Input: part model. Units: mm. Frame: model coordinates. A direction names the side the tool comes from. Give positions to 0.01 mm unless a question says otherwise; leave off trailing zeros. Order: outer loops, then holes, each group sorted by start corner. A loop starts at its lowest first (then second) coordinate and runs counter-clockwise, first axis right, second up. Notation, with made-up numbers: (-20.75, 75) - (16.25, 75) arc R33 cw to (16.25, 104) - close; hole circle Ø11 at (55, -38). An arc over 180 degrees is marked (long way). Answer in a Markdown table with one row per item. Add a question column.
1. Ray query, line 1 (Y direction, x = 90.5, z = 0.55); line 2 (X direction, y = 67.5, z = 0.6); line 3 (X direction, y = 45, z = 5.5). Return the intervals inside material, ascending. Write a range as [from, to].
2. Access query for faces 5 (the face through (46, 9.5, 6)), 6 (the face through (7.5, 35, 6)), 7 (the face through (85.5, 35, 6)), 8 (the face through (40, 3.6, -4)), 9 (the face through (65, 2, -4)). Directions: +Z, -Z, +X, -X, +Y, -Y. A direction counts if a zero-diameter tool reaches every point of the face in a straight line with its end or side. Return the directions, or none.
3. Section query C-C on x = 81. Return loops of the section in (y, z).
4. Contact query for flat-ended pins moving along their axis: pin 1 (5 mm diameter, centred on x = 2.5, y = 2.5, fed in from +Z); pin 2 (2.5 mm diameter, centred on x = 51.5, z = -3.5, fed in from +Y); pin 3 (1.5 mm diameter, centred on x = 79.5, y = 33.5, fed in from -Z); pin 4 (9 mm diameter, centred on x = 35, z = -3.5, fed in from -Y). Output: stop coordinate, or through.
5. Mould query, pull axis X, two halves, no side actions, for faces 1 (the face through (14, 2, -4)), 2 (the face through (40, 1.4, -4)), 3 (the face through (3.306, 68.765, 0.811)), 4 (the face through (40, 3, -8)). Classes: released by +X, released by -X, zero draft, split by the parting line, or undercut.
6. Section query D-D on y = 8. Return loops of the section in (x, z), and give its area (3 significant figures).
7. Section query A-A on x = 90.5. Return loops of the section in (y, z).
8. Section query B-B on y = 40. Return loops of the section in (x, z).
```python
from build123d import *

# Parameters (mm, degrees)
SKETCH_1_W          = 93
SKETCH_1_H          = 70
EXTRUDE_1_DEPTH     = 1.6
SKETCH_2_R          = 1.5
CUT_EXTRUDE_1_DEPTH = 117.411167849
SKETCH_3_W          = 78
SKETCH_3_H          = 51
EXTRUDE_2_DEPTH     = 9
SKETCH_4_W          = 51
SKETCH_4_H          = 2.2
EXTRUDE_3_DEPTH     = 8
SKETCH_5_R          = 0.4
EXTRUDE_4_DEPTH     = 2


with BuildPart() as part:
    # 草图1 → 凸台-拉伸1 (new body)
    with BuildSketch(Plane.XY):
        with Locations((46.5, 35)):
            Rectangle(SKETCH_1_W, SKETCH_1_H)
    extrude(amount=EXTRUDE_1_DEPTH)

    # 草图2 → 切除-拉伸1 (cut, through all)
    with BuildSketch(Plane.XY.offset(1.6)):
        with Locations((2.5, 2.5)):
            Circle(SKETCH_2_R)
        with Locations((90.5, 2.5)):
            Circle(SKETCH_2_R)
        with Locations((90.5, 67.5)):
            Circle(SKETCH_2_R)
        with Locations((2.5, 67.5)):
            Circle(SKETCH_2_R)
    extrude(amount=-CUT_EXTRUDE_1_DEPTH, mode=Mode.SUBTRACT)

    # 草图3 → 凸台-拉伸2 (add)
    with BuildSketch(Plane.XY.offset(1.6)):
        with Locations((46.5, 35)):
            Rectangle(SKETCH_3_W, SKETCH_3_H)
    extrude(amount=EXTRUDE_2_DEPTH)

    # 草图4 → 凸台-拉伸3 (add)
    with BuildSketch(Plane(origin=(0, 0, 0), x_dir=(-1, 0, 0), z_dir=(0, 0, -1))):
        with Locations((-39.5, 2.5)):
            Rectangle(SKETCH_4_W, SKETCH_4_H)
    extrude(amount=EXTRUDE_3_DEPTH)

    # 草图5 → 凸台-拉伸4 (add)
    with BuildSketch(Plane(origin=(0, 0, -8), x_dir=(-1, 0, 0), z_dir=(0, 0, -1))):
        with Locations(Location((-38.23, 2.5, 0), (0, 0, 180))):
            Circle(SKETCH_5_R)
        with Locations(Location((-40.77, 2.5, 0), (0, 0, 180))):
            Circle(SKETCH_5_R)
        with Locations(Location((-43.31, 2.5, 0), (0, 0, 180))):
            Circle(SKETCH_5_R)
        with Locations(Location((-45.85, 2.5, 0), (0, 0, 180))):
            Circle(SKETCH_5_R)
        with Locations(Location((-48.39, 2.5, 0), (0, 0, 180))):
            Circle(SKETCH_5_R)
        with Locations(Location((-50.93, 2.5, 0), (0, 0, 180))):
            Circle(SKETCH_5_R)
        with Locations(Location((-53.47, 2.5, 0), (0, 0, 180))):
            Circle(SKETCH_5_R)
        with Locations(Location((-56.01, 2.5, 0), (0, 0, 180))):
            Circle(SKETCH_5_R)
        with Locations(Location((-58.55, 2.5, 0), (0, 0, 180))):
            Circle(SKETCH_5_R)
        with Locations(Location((-61.09, 2.5, 0), (0, 0, 180))):
            Circle(SKETCH_5_R)
        with Locations(Location((-63.63, 2.5, 0), (0, 0, 180))):
            Circle(SKETCH_5_R)
        with Locations(Location((-35.69, 2.5, 0), (0, 0, 180))):
            Circle(SKETCH_5_R)
        with Locations(Location((-33.15, 2.5, 0), (0, 0, 180))):
            Circle(SKETCH_5_R)
        with Locations(Location((-30.61, 2.5, 0), (0, 0, 180))):
            Circle(SKETCH_5_R)
        with Locations(Location((-28.07, 2.5, 0), (0, 0, 180))):
            Circle(SKETCH_5_R)
        with Locations(Location((-25.53, 2.5, 0), (0, 0, 180))):
            Circle(SKETCH_5_R)
        with Locations(Location((-22.99, 2.5, 0), (0, 0, 180))):
            Circle(SKETCH_5_R)
        with Locations(Location((-20.45, 2.5, 0), (0, 0, 180))):
            Circle(SKETCH_5_R)
        with Locations(Location((-17.91, 2.5, 0), (0, 0, 180))):
            Circle(SKETCH_5_R)
        with Locations(Location((-15.37, 2.5, 0), (0, 0, 180))):
            Circle(SKETCH_5_R)
    extrude(amount=EXTRUDE_4_DEPTH)


solid = part.part
```
Answer:
| question | item | result |
|---|---|---|
| 1 | line 1 | y = [0, 1], [4, 66], [69, 70] |
| 1 | line 2 | x = [0, 1], [4, 89], [92, 93] |
| 1 | line 3 | x = [7.5, 85.5] |
| 2 | face 5 | +Z, +X, -X, -Y |
| 2 | face 6 | +Z, -X, +Y, -Y |
| 2 | face 7 | +Z, +X, +Y, -Y |
| 2 | face 8 | -Z, +X, -X, +Y |
| 2 | face 9 | -Z, +X, +Y, -Y |
| 3 | outline | (0, 0) - (70, 0) - (70, 1.6) - (60.5, 1.6) - (60.5, 10.6) - (9.5, 10.6) - (9.5, 1.6) - (0, 1.6) - close |
| 4 | pin 1 | stops at z = 1.6 |
| 4 | pin 2 | stops at y = 3.6 |
| 4 | pin 3 | stops at z = 0 |
| 4 | pin 4 | stops at y = 0 |
| 5 | face 1 | released by -X |
| 5 | face 2 | zero draft |
| 5 | face 3 | undercut |
| 5 | face 4 | undercut |
| 6 | outline | (0, 0) - (93, 0) - (93, 1.6) - (0, 1.6) - close |
| 6 | area | 149 mm² |
| 7 | outline | (0, 0) - (1, 0) - (1, 1.6) - (0, 1.6) - close; (4, 0) - (66, 0) - (66, 1.6) - (4, 1.6) - close; (69, 0) - (70, 0) - (70, 1.6) - (69, 1.6) - close |
| 8 | outline | (0, 0) - (93, 0) - (93, 1.6) - (85.5, 1.6) - (85.5, 10.6) - (7.5, 10.6) - (7.5, 1.6) - (0, 1.6) - close |
